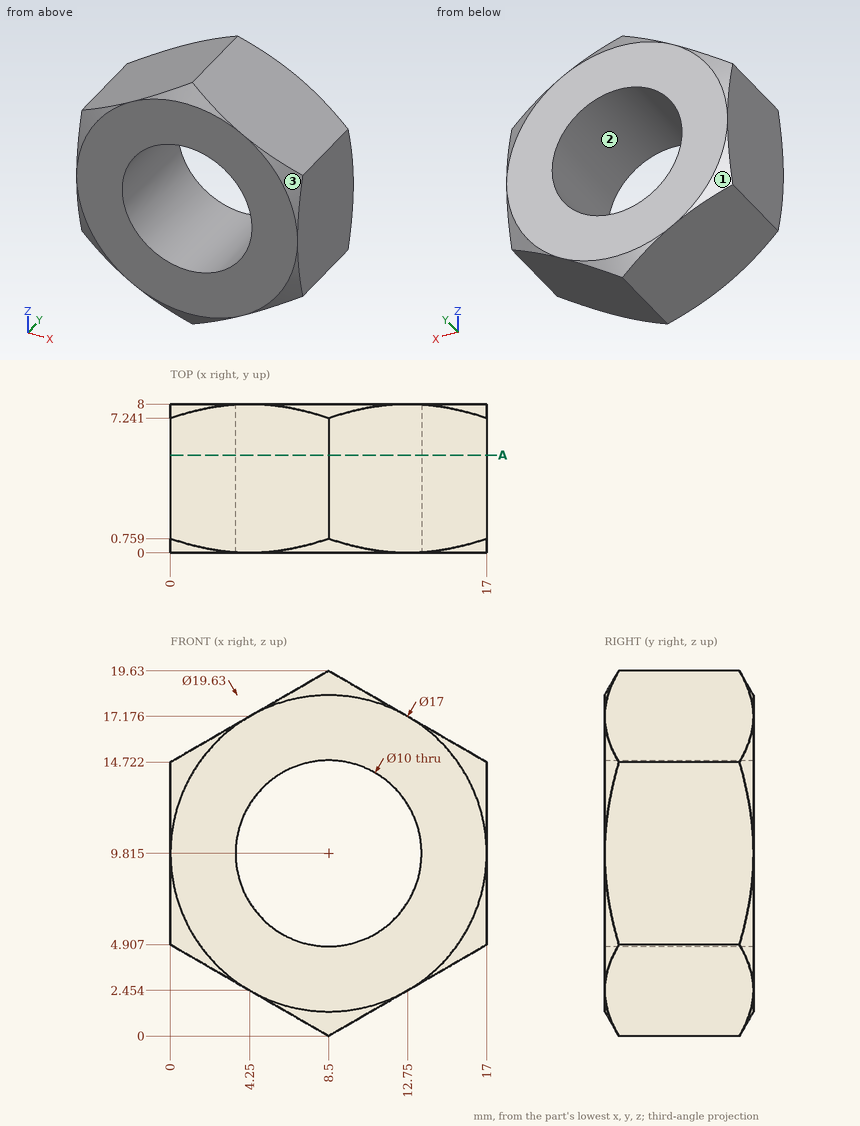
For this review, use the dimensioned drawing (mm, ordinates from the lowest corner) and the shaded views. Round coordinates to 2 decimals unless told otherwise and drop trailing zeros. Write each loop counter-clockwise with the first axis right and the second up, starting at its lowest first coordinate (ties: lowest second). Pieces come first, ordered by that corner, then holes. Notation, with made-up numbers: (70, 46) -> (129, 46) arc R12 ccw to (129, 58) -> close; hole circle Ø11 at (23, -1.75). An arc over 180 degrees is marked (long way). One line per item, written item: value. Start each with the question number.
Q1. The part is to be moulded in two halves that separate along X. For the marked faces 1, 2 and 3, say which applies: pulls with the +X half, pulls with the -X half, needs draft (parallel to the pull), parting line crosses it, or undercut.
Q2. Add section A-A (y = 5.25). Give the boundary of the cut face in (x, z) (1 decimal), then the cut area to 3 significant figures.
Q3. Insertion check: P1, Ø1.5, axis at x = 14.5, z = 2.5, coming from the +Y side. The pin has a flat end and moves straight along its axis. Give the tip position at first contact, or say it passes through.
Q4. To check wall thickness, follow probe 1 along Z at (x, y) = (6, 6.75) (1 decimal); probe 2 along Z at (x, y) = (11.5, 7.5) (1 decimal); probe 3 along X at (y, z) = (3.75, 7.5). State the ranges of each line that lie inside material, in increasing order.
Response:
1. face 1: pulls with the -X half
1. face 2: undercut
1. face 3: pulls with the +X half
2. outline: (0, 4.9) -> (8.5, 0) -> (17, 4.9) -> (17, 14.7) -> (8.5, 19.6) -> (0, 14.7) -> close; hole circle Ø10 at (8.5, 9.8)
2. area: 172 mm^2
3. P1: passes through
4. probe 1: z = 1.4 to 5.5, 14.1 to 18.2
4. probe 2: z = 1.7 to 5.8, 13.8 to 17.9
4. probe 3: x = 0 to 4.07, 12.93 to 17
